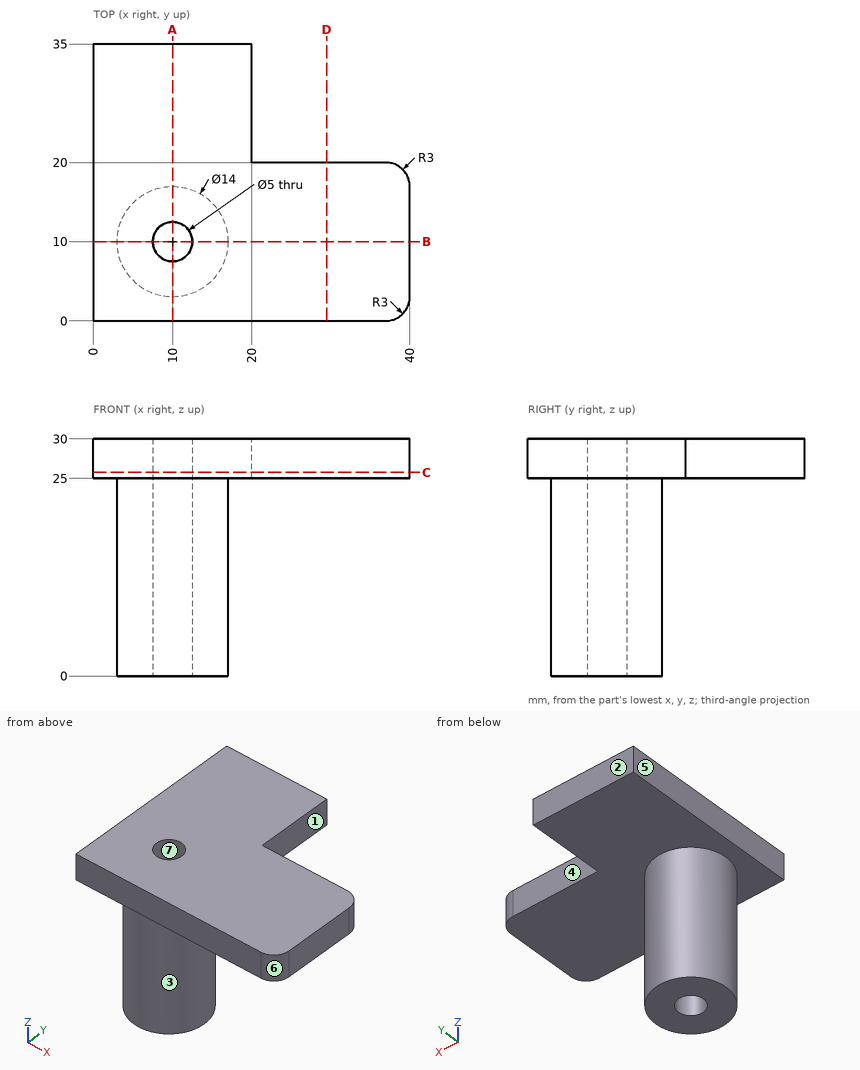
Design review of the part shown in the three views and the two pictorial views. Dimensions are in mm from the part's minimum x, y and z. A direction names the side the tool comes from. Give positions to 0.01 mm unless a question says otherwise; leave off trailing zeros. Loops run counter-clockwise (first coordinate to the right, second up) from the corner with the lowest first, then second, coordinate; pieces in that order, holes last. Notation, with made-up numbers: M 51.25,37.5 L 110.25,37.5 A8 ccw 110.25,51.5 Z; hole C 54.25,17 d11. An arc over 180 degrees is marked long. Answer as a JSON object with one key per item and string values.
Item 1: We need section B-B (y = 10). State the section outline as (x, z) points.
Output values:
{"outline": "M 0,25 L 3,25 L 3,0 L 7.5,0 L 7.5,30 L 0,30 Z; M 12.5,0 L 17,0 L 17,25 L 40,25 L 40,30 L 12.5,30 Z"}
Item 2: We need section D-D (x = 29.5). State the section outline as (y, z) points, and give its area (3 significant figures).
Output values:
{"outline": "M 0,25 L 20,25 L 20,30 L 0,30 Z", "area": "100 mm2"}
Item 3: Machinability: for the marked faces 1, 2 and 3, which of the approach directions +Z, -Z, +X, -X, +Y, -Y give a long, thin tool a straight path to every point of the face, cutting with its end or side? Answer none if there is none.
Output values:
{"face 1": "+Z, -Z, +X, +Y", "face 2": "+Z, -Z, +X, -X, +Y", "face 3": "-Z"}
Item 4: We need section C-C (z = 25.75). State the section outline as (x, y) points, and give its area (3 significant figures).
Output values:
{"outline": "M 0,0 L 37,0 A3 ccw 40,3 L 40,17 A3 ccw 37,20 L 20,20 L 20,35 L 0,35 Z; hole C 10,10 d5", "area": "1,080 mm2"}
Item 5: Wall thickness on line 1 along X through (y, z) = (10, 15); line 2 along Y through (x, z) = (24, 26.25): over which ranges is each line inside the solid? List them lowest first.
Output values:
{"line 1": "x = 3 to 7.5, 12.5 to 17", "line 2": "y = 0 to 20"}
Item 6: Mouldability with a two-part tool opening along X and no side actions: class the marked faces 4, 5, 6 and 7 as pulls with the +X half, pulls with the -X half, needs draft (parallel to the pull), parting line crosses it, or undercut.
Output values:
{"face 4": "needs draft", "face 5": "pulls with the -X half", "face 6": "pulls with the +X half", "face 7": "undercut"}
Item 7: We need section A-A (x = 10). State the section outline as (y, z) points.
Output values:
{"outline": "M 0,25 L 3,25 L 3,0 L 7.5,0 L 7.5,30 L 0,30 Z; M 12.5,0 L 17,0 L 17,25 L 35,25 L 35,30 L 12.5,30 Z"}
Item 8: For P1, Ø1.5, axis at x = 28, z = 27.5, coming from the +Y side; P2, Ø4, axis at x = 16, z = 18, coming from the -Y side; P3, Ø1.5, axis at x = 34.5, y = 21, coming from the -Z side; P4, Ø1, axis at x = 13, y = 17.5, coming from the -Z side, all flat-tipped, find the tip position at first contact; note any pin that passes through.
Output values:
{"P1": "stops at y = 20", "P2": "stops at y = 4.26", "P3": "passes through", "P4": "stops at z = 25"}
